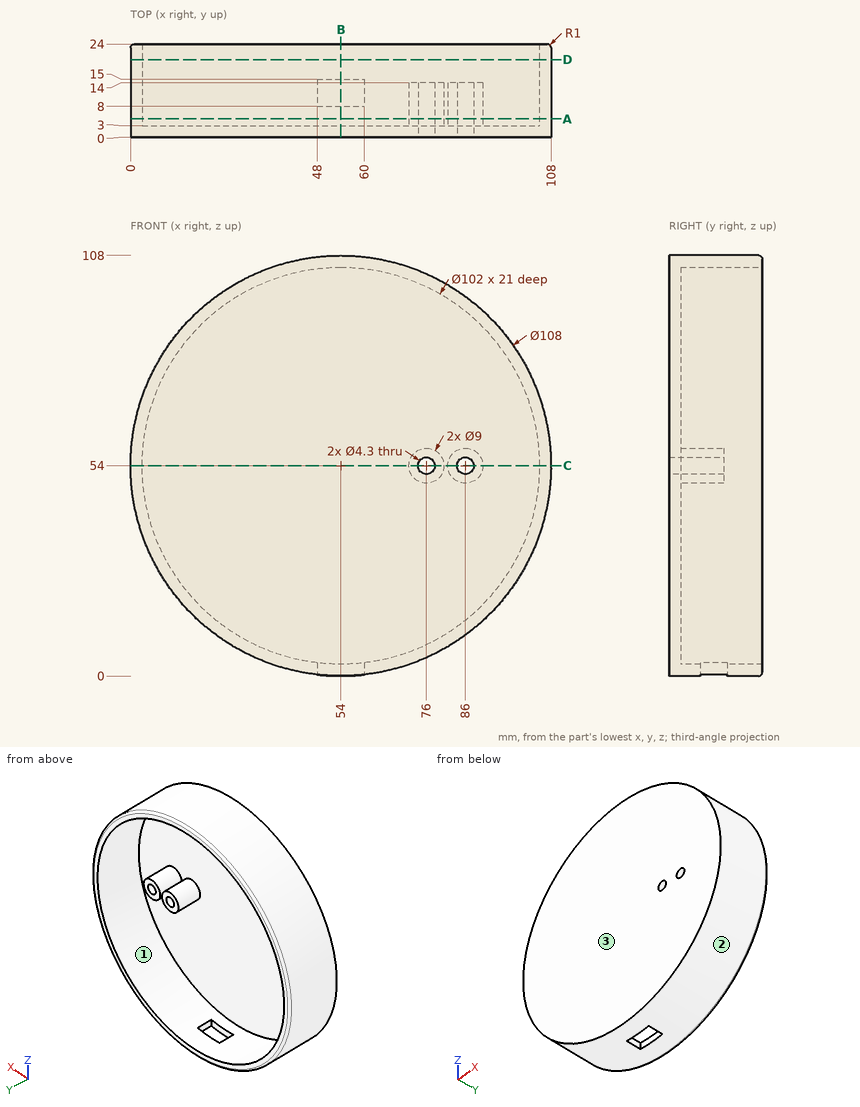
Can you work these out from the drawing? Everything is in mm from the part's minimum corner. Give positions to 0.01 mm unless a question says otherwise; leave off trailing zeros. Loops run counter-clockwise (first coordinate to the right, second up) from the corner with the lowest first, then second, coordinate; pieces in that order, holes last. Notation, with made-up numbers: (62, 65.5) -> (86, 65.5) arc R15 ccw to (86, 84.5) -> close; hole circle Ø7 at (85, 17.5). An arc over 180 degrees is marked (long way). Put each result on its own line as item: value.
(1) Imagine slicing it at C-C on z = 54. Write out the boundary of the cut face in (x, y).
Computed:
outline: (0, 0) -> (73.85, 0) -> (73.85, 14) -> (71.5, 14) -> (71.5, 3) -> (3, 3) -> (3, 24) -> (1, 24) arc R1 ccw to (0, 23) -> close; (78.15, 0) -> (83.85, 0) -> (83.85, 14) -> (81.5, 14) -> (81.5, 3) -> (80.5, 3) -> (80.5, 14) -> (78.15, 14) -> close; (88.15, 0) -> (108, 0) -> (108, 23) arc R1 ccw to (107, 24) -> (105, 24) -> (105, 3) -> (90.5, 3) -> (90.5, 14) -> (88.15, 14) -> close
(2) I'm going to push flat-ended pins straight in: pin 1 Ø7 at (x, z) = (87.5, 54) entering from +Y; pin 2 Ø1.5 at (x, y) = (88, 16) entering from -Z; pin 3 Ø5 at (x, z) = (66.5, 42) entering from +Y. Where does each tip first touch, or does it pass through?
Computed:
pin 1: y = 14
pin 2: z = 11.45
pin 3: y = 3
(3) Please list where these lines run through material, in increasing order: probe 1 along X at (y, z) = (7.75, 54); probe 2 along Z at (x, y) = (86, 8.5); probe 3 along Z at (x, y) = (76, 10.5). Write a range as [from, to].
Computed:
probe 1: [0, 3], [71.5, 73.85], [78.15, 80.5], [81.5, 83.85], [88.15, 90.5], [105, 108]
probe 2: [10.5, 14.29], [49.5, 51.85], [56.15, 58.5], [93.71, 97.5]
probe 3: [4.68, 7.99], [49.5, 51.85], [56.15, 58.5], [100.01, 103.32]
(4) Imagine slicing it at B-B on x = 54. Write out the boundary of the cut face in (y, z).
Computed:
outline: (0, 0) -> (8, 0) -> (8, 3) -> (3, 3) -> (3, 105) -> (24, 105) -> (24, 107) arc R1 ccw to (23, 108) -> (0, 108) -> close; (15, 0) -> (23, 0) arc R1 ccw to (24, 1) -> (24, 3) -> (15, 3) -> close
(5) Imagine slicing it at A-A on y = 4.75. Write out the boundary of the cut face in (x, z), plus the area to 3 significant figures.
Computed:
outline: circle Ø108 at (54, 54); circle Ø9 at (76, 54); circle Ø9 at (86, 54); hole circle Ø102 at (54, 54); hole circle Ø4.3 at (76, 54); hole circle Ø4.3 at (86, 54)
area: 1,090 mm^2
(6) Thinking about a two-plate mould opening in Z: for the marked faces 1, 2 and 3, which applies, pulls with the +Z half, pulls with the -Z half, needs draft (parallel to the pull), parting line crosses it, or undercut?
Computed:
face 1: undercut
face 2: parting line crosses it
face 3: needs draft
(7) Imagine slicing it at D-D on y = 20. Write out the boundary of the cut face in (x, z), plus the area to 3 significant figures.
Computed:
outline: circle Ø108 at (54, 54); hole circle Ø102 at (54, 54)
area: 990 mm^2
